Answer from the drawing. Dimensions are ordinates in mm from the lowest x, y and z of the part. Round coordinates to 2 decimals unless told otherwise and drop trailing zeros. Loops run counter-clockwise (first coordinate to the right, second up) from the corner with the lowest first, then second, coordinate; pieces in that order, holes last. Notation, with made-up numbers: (39, 72.25) -> (50, 72.25) arc R15 ccw to (50, 101.25) -> close; hole circle Ø8 at (17.25, 61). An arc over 180 degrees is marked (long way). Use CSV: the item, a comma, the result in double quotes. Start each with the question number.
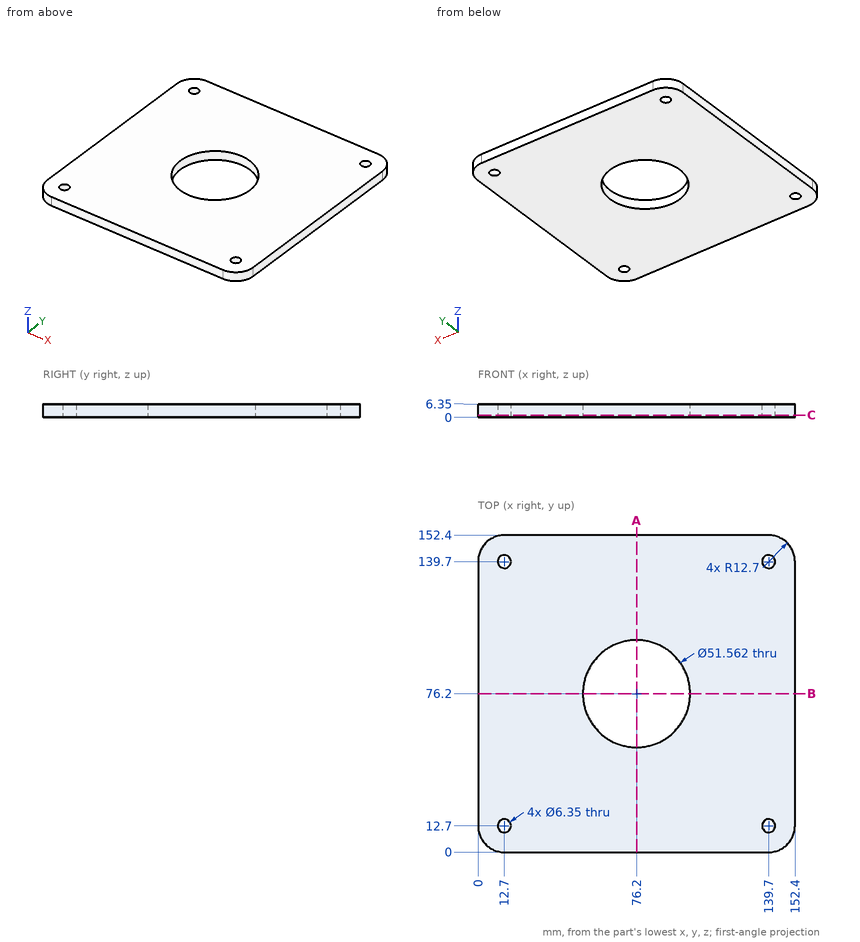
Q1. Straight lines are drawn through the part: line 1 (Y direction, x = 139.7, z = 5) (3 decimals); line 2 (Y direction, x = 76.2, z = 3.5); line 3 (X direction, y = 142.5, z = 5.25). For each, find the intervals that lie inside material, in ascending order. Write a range as from..to.
Q2. Section C-C, the plane z = 1 is taken. Write down the section's boundary in (x, y) (3 decimals).
Q3. Section A-A, the plane x = 76.2 is taken. Write down the section's boundary in (y, z).
Q4. Each of these flat-tipped pins is pushed along its axis until it touches: pin 1 (7.5 mm diameter, centred on x = 139.7, y = 12.7, fed in from -Z); pin 2 (5.5 mm diameter, centred on x = 139.7, y = 139.7, fed in from -Z). Where does it stop, or does it pass through?
Report:
1,line 1,"y = 0..9.525, 15.875..136.525, 142.875..152.4"
1,line 2,"y = 0..50.42, 101.98..152.4"
1,line 3,"x = 0.31..11.2, 14.2..138.2, 141.2..152.09"
2,outline,"(0, 12.7) arc R12.7 ccw to (12.7, 0) -> (139.7, 0) arc R12.7 ccw to (152.4, 12.7) -> (152.4, 139.7) arc R12.7 ccw to (139.7, 152.4) -> (12.7, 152.4) arc R12.7 ccw to (0, 139.7) -> close; hole circle Ø6.35 at (12.7, 12.7); hole circle Ø6.35 at (12.7, 139.7); hole circle Ø51.562 at (76.2, 76.2); hole circle Ø6.35 at (139.7, 12.7); hole circle Ø6.35 at (139.7, 139.7)"
3,outline,"(0, 0) -> (50.42, 0) -> (50.42, 6.35) -> (0, 6.35) -> close; (101.98, 0) -> (152.4, 0) -> (152.4, 6.35) -> (101.98, 6.35) -> close"
4,pin 1,"stops at z = 0"
4,pin 2,"passes through"
